Geometry check sheet. Reference: the model listing, model coordinates, mm. A direction names the side the tool comes from. Round coordinates to 2 decimals unless told otherwise and drop trailing zeros. Order: outer loops, then holes, each group sorted by start corner. A loop starts at its lowest first (then second) coordinate and runs counter-clockwise, first axis right, second up. Notation, with made-up numbers: (78, -1.75) - (85, -1.75) arc R19 ccw to (85, 2.25) - close; hole circle Ø4 at (54.25, -9.75). An arc over 180 degrees is marked (long way). Use a Markdown table: item, result. Add a question column.
(1) Section check C-C on y = 25.5. Record the boundary of the cut face in (x, z), then the cut area to 3 significant figures.
(2) Section check D-D on x = 76. Record the boundary of the cut face in (y, z), then the cut area to 3 significant figures.
(3) Mould release check, pull along X, two halves, no side actions. Record for faces 1 (the face through (56.494, 51, 6)), 2 (the face through (58.012, 61.417, 10.477)), 3 (the face through (0, 51, 1)), 4 (the face through (72, 51, 3)): released by +X, released by -X, zero draft, split by the parting line, or undercut.
(4) Section check B-B on y = 61.5. Record the boundary of the cut face in (x, z).
(5) Access from +Z, -Z, +X, -X, +Y, -Y to the whole of each face (thin tool, end or side, straight path). Record for faces 5 (the face through (56.268, 8, 8)), 6 (the face through (50, 10.006, 6)), 7 (the face through (51, 51, 0)).
(6) Section check A-A on x = 50. Record the boundary of the cut face in (y, z), then the cut area to 3 significant figures.
(7) Gauge pin test, flat ends, axial feed: P1, Ø0.5, axis at x = 50, z = 3.5, coming from the +Y side; P2, Ø1, axis at x = 19, y = 59.5, coming from the -Z side; P3, Ø12, axis at x = 78.5, y = 21, coming from the +Z side. Record the tip position at first contact, or that the pin passes through.
(8) Thickness scan on line 1 along Y through (x, z) = (37, -0.75); line 2 along X through (y, z) = (53.5, 8.5); line 3 along Z through (x, y) = (20.5, 69.5). Record the ranges inside material, lowest first. Write a range as [from, to].
Autodesk Inventor part; units mm, degrees
ref_plane "YZ Plane" through (0, 0, 0) normal (1, 0, 0) x (0, 1, 0)
ref_plane "XZ Plane" through (0, 0, 0) normal (0, 1, 0) x (-1, 0, 0)
ref_plane "XY Plane" through (0, 0, 0) normal (0, 0, 1) x (1, 0, 0)
sketch "Sketch1" plane through (0, 0, 0) normal (0, 0, 1) x (1, 0, 0)
  line L0 (0, 0) -> (100, 0)
  line L1 (100, 0) -> (100, 100)
  line L2 (100, 100) -> (0, 100)
  line L3 (0, 100) -> (0, 0)
  dimension "d0" = 100
  dimension "d1" = 100
extrude "Extrusion1" add sketch "Sketch1" along normal blind 3
sketch "Sketch2" plane through (0, 0, 3) normal (0, 0, 1) x (1, 0, 0)
  line L0 (36, 97.5) -> (64, 97.5)
  line L1 (64, 97.5) -> (64, 2.5)
  line L2 (64, 2.5) -> (36, 2.5)
  line L3 (36, 2.5) -> (36, 97.5)
  line L4 (0, 0) -> (100, 0)
  line L5 (0, 100) -> (0, 0)
  dimension "d6" = 28
  dimension "d7" = 95
  dimension "d8" = 2.5
  dimension "d9" = 36
extrude "Extrusion2" add sketch "Sketch2" along normal blind 13 draft -30
sketch "Sketch4" plane through (0, 0, 16) normal (0, 0, 1) x (1, 0, 0)
  line L0 (43.5056, 10.0056) -> (43.5056, 89.9944)
  line L1 (56.4944, 10.0056) -> (43.5056, 10.0056)
  line L2 (56.4944, 89.9944) -> (56.4944, 10.0056)
  line L3 (43.5056, 89.9944) -> (56.4944, 89.9944)
  point P0 (0, 0)
extrude "Extrusion3" cut sketch "Sketch4" against normal blind 13
sketch "Sketch5" plane through (0, 0, 0) normal (0, -1, 0) x (1, 0, 0)
  line L0 (56.4944, 16) -> (43.5056, 16)
  line L1 (43.5056, 16) -> (56.4944, 16)
  line L2 (56.2684, 16) -> (67.0318, 16)
  line L3 (67.0318, 16) -> (67.0318, 7)
  line L4 (67.0318, 7) -> (56.2684, 7)
  line L5 (56.2684, 7) -> (56.2684, 16)
  point P0 (0, 0)
  dimension "d14" = 9
fillet "Fillet1" radius 2 4 edges at (50, 10.0056, 16) (56.4944, 50, 16) (43.5056, 50, 16) (50, 89.9944, 16)
extrude "Extrusion4" cut sketch "Sketch5" against normal blind 30
sketch "Sketch6" plane through (0, 0, 0) normal (0, 0, -1) x (-1, 0, 0)
  line L0 (-100, 100) -> (0, 100)
  line L1 (0, 0) -> (-100, 0)
  line L2 (-100, 100) -> (0, 100)
  line L3 (0, 100) -> (0, 0)
  line L4 (0, 0) -> (-100, 0)
  line L5 (-100, 0) -> (-100, 100)
extrude "Extrusion5" add sketch "Sketch6" along normal blind 2
sketch "Sketch7" plane through (0, 0, -2) normal (0, 0, -1) x (-1, 0, 0)
  line L0 (-98, 98) -> (-2, 98)
  line L1 (-2, 98) -> (-2, 2)
  line L2 (-2, 2) -> (-98, 2)
  line L3 (-98, 2) -> (-98, 98)
  line L4 (0, 100) -> (-100, 100)
  line L5 (-100, 100) -> (-100, 0)
  line L6 (-100, 0) -> (0, 0)
  line L7 (0, 0) -> (0, 100)
  dimension "d19" = 2
  dimension "d20" = 2
  dimension "d21" = 2
  dimension "d22" = 2
extrude "Extrusion6" cut sketch "Sketch7" against normal blind 2 contours L0 L1 L2 L3
sketch "Sketch8" plane through (0, 0, 3) normal (0, 0, 1) x (1, 0, 0)
  line L0 (48.5, 51.5) -> (51.5, 51.5)
  line L1 (51.5, 51.5) -> (51.5, 48.5)
  line L2 (51.5, 48.5) -> (48.5, 48.5)
  line L3 (48.5, 48.5) -> (48.5, 51.5)
  line L4 (0, 100) -> (0, 0)
  line L5 (100, 100) -> (0, 100)
  dimension "d25" = 3
  dimension "d26" = 3
  dimension "d27" = 48.5
  dimension "d28" = 48.5
extrude "Extrusion7" add sketch "Sketch8" along normal blind 1
properties part number "Weight_Plate"
Check sheet entries:
| question | item | result |
|---|---|---|
| 1 | outline | (0, -2) - (2, -2) - (2, 0) - (98, 0) - (98, -2) - (100, -2) - (100, 3) - (64, 3) - (61.69, 7) - (56.49, 7) - (56.49, 3) - (43.51, 3) - (43.51, 8.54) arc R2 ccw to (39.77, 9.54) - (36, 3) - (0, 3) - close |
| 1 | area | 372 mm2 |
| 2 | outline | (0, -2) - (2, -2) - (2, 0) - (98, 0) - (98, -2) - (100, -2) - (100, 3) - (0, 3) - close |
| 2 | area | 308 mm2 |
| 3 | face 1 | undercut |
| 3 | face 2 | undercut |
| 3 | face 3 | released by -X |
| 3 | face 4 | zero draft |
| 4 | outline | (0, -2) - (2, -2) - (2, 0) - (98, 0) - (98, -2) - (100, -2) - (100, 3) - (64, 3) - (60.23, 9.54) arc R2 ccw to (56.49, 8.54) - (56.49, 3) - (43.51, 3) - (43.51, 8.54) arc R2 ccw to (39.77, 9.54) - (36, 3) - (0, 3) - close |
| 5 | face 5 | +Z, +X, -Y |
| 5 | face 6 | +Z |
| 5 | face 7 | -Z |
| 6 | outline | (0, -2) - (2, -2) - (2, 0) - (98, 0) - (98, -2) - (100, -2) - (100, 3) - (97.5, 3) - (93.73, 9.54) arc R2 ccw to (89.99, 8.54) - (89.99, 3) - (51.5, 3) - (51.5, 4) - (48.5, 4) - (48.5, 3) - (10.01, 3) - (10.01, 8.54) arc R2 ccw to (6.27, 9.54) - (2.5, 3) - (0, 3) - close |
| 6 | area | 389 mm2 |
| 7 | P1 | stops at y = 97.36 |
| 7 | P2 | stops at z = 0 |
| 7 | P3 | stops at z = 3 |
| 8 | line 1 | y = [0, 2], [98, 100] |
| 8 | line 2 | x = [39.18, 43.51], [56.49, 60.82] |
| 8 | line 3 | z = [0, 3] |
